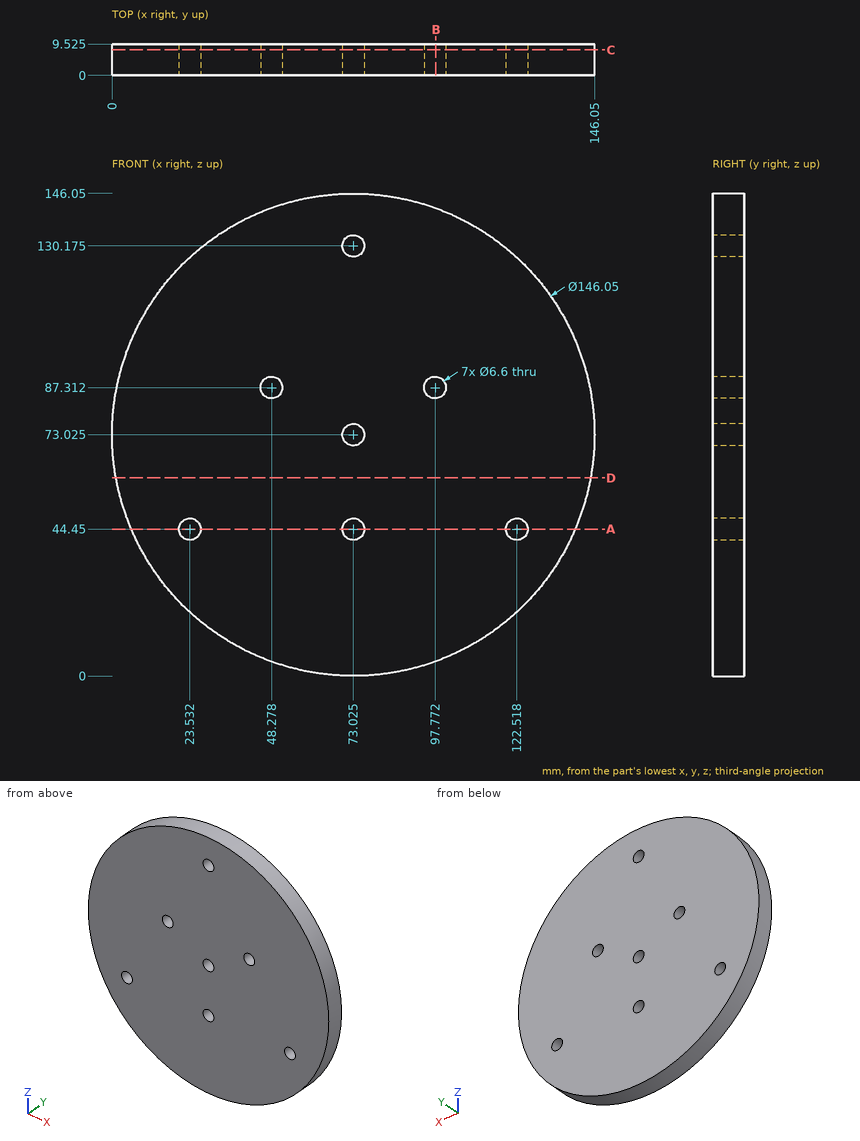
Job drawing, mm, ordinate dimensions from the low corner. One solid piece. Coordinates: 2 decimals unless noted, no trailing zeros. Loops run counter-clockwise (first coordinate to the right, second up) from the corner with the lowest first, then second, coordinate; pieces in that order, holes last. Notation, with made-up numbers: (30.25, 71) -> (88.25, 71) arc R14 cw to (88.25, 90) -> close; hole circle Ø11 at (41, 63). An arc over 180 degrees is marked (long way). One line per item, written item: value.
1. Slice it at B-B on x = 98. Write the cut outline in (y, z) (1 decimal), and give its area (3 significant figures).
Answers:
outline: (0, 4.4) -> (9.5, 4.4) -> (9.5, 84) -> (0, 84) -> close; (0, 90.6) -> (9.5, 90.6) -> (9.5, 141.6) -> (0, 141.6) -> close
area: 1,240 mm^2
2. Flat gauge pins, fed straight in: P1, Ø4, axis at x = 56, y = 1, coming from the +Z side; P2, Ø7.5, axis at x = 73.025, z = 44.45, coming from the -Y side; P3, Ø2, axis at x = 99.5, y = 4, coming from the -Z side; P4, Ø1.5, axis at x = 39.5, y = 7.5, coming from the -Z side. Where does each tip first touch, or does it go through?
Answers:
P1: stops at z = 144.49
P2: stops at y = 0
P3: stops at z = 4.59
P4: stops at z = 7.77
3. Slice it at D-D on z = 60. Write the cut outline in (x, y) (1 decimal).
Answers:
outline: (1.2, 0) -> (144.9, 0) -> (144.9, 9.5) -> (1.2, 9.5) -> close
4. Slice it at C-C on y = 7.75. Give the number of separate pieces and of enclosed holes in the cut face, and give its area (3 significant figures).
Answers:
separate pieces: 1
enclosed holes: 7
area: 16,500 mm^2
5. Drill centre lines: line 1 (Z direction, x = 74, y = 6.5) (1 decimal); line 2 (X direction, y = 4, z = 44.45) (1 decimal); line 3 (Z direction, x = 25, y = 3.5) (1 decimal). Where is each one in solid material? Low to high. Write a range as [from, to].
Answers:
line 1: z = [0, 41.3], [47.6, 69.9], [76.2, 127], [133.3, 146]
line 2: x = [5.8, 20.2], [26.8, 69.7], [76.3, 119.2], [125.8, 140.2]
line 3: z = [18, 41.5], [47.4, 128]
6. Slice it at A-A on z = 44.45. Write the cut outline in (x, y) (1 decimal).
Answers:
outline: (5.8, 0) -> (20.2, 0) -> (20.2, 9.5) -> (5.8, 9.5) -> close; (26.8, 0) -> (69.7, 0) -> (69.7, 9.5) -> (26.8, 9.5) -> close; (76.3, 0) -> (119.2, 0) -> (119.2, 9.5) -> (76.3, 9.5) -> close; (125.8, 0) -> (140.2, 0) -> (140.2, 9.5) -> (125.8, 9.5) -> close
